```python
from build123d import *

# Parameters (mm, degrees)
SKETCH1_R           = 41.148
BOSS_EXTRUDE1_DEPTH = 38.1
SKETCH2_R           = 3.18135
CUT_EXTRUDE1_DEPTH  = 29.464
CIRPATTERN1_COUNT   = 6
SKETCH3_R           = 44.45
SKETCH3_R_2         = 41.148
BOSS_EXTRUDE2_DEPTH = 57.15
FILLET1_R           = 12.7
CHAMFER1_SIZE       = 1.27
CHAMFER1_SIZE2      = 0.592210726


with BuildPart() as part:
    # Sketch1 → Boss-Extrude1 (new body)
    with BuildSketch(Plane(origin=(0, 0, 0), x_dir=(1, 0, 0), z_dir=(0, 1, 0))):
        Polygon((0, -58.65878735), (50.8, -29.329393675), (50.8, 29.329393675), (0, 58.65878735), (-50.8, 29.329393675), (-50.8, -29.329393675), align=None)
        with Locations(Location((0, 0, 0), (0, 0, 90))):
            Circle(SKETCH1_R, mode=Mode.SUBTRACT)
    extrude(amount=BOSS_EXTRUDE1_DEPTH)

    # Sketch2 → Cut-Extrude1 (cut)
    with BuildSketch(Plane.ZY.offset(50.8)):
        with Locations((0, 19.05)):
            Circle(SKETCH2_R)
    cut_extrude1 = extrude(amount=-CUT_EXTRUDE1_DEPTH, mode=Mode.SUBTRACT)

    # CirPattern1: Cut-Extrude1 ×6 about axis
    cirpattern1_axis = Axis((0, 38.1, 0), (0, 1, 0))
    for i in range(1, CIRPATTERN1_COUNT):
        add(cut_extrude1.rotate(cirpattern1_axis, i * 360 / CIRPATTERN1_COUNT), mode=Mode.SUBTRACT)

    # Sketch3 → Boss-Extrude2 (add)
    with BuildSketch(Plane(origin=(-50.8, 38.1, -29.329393675), x_dir=(1, 0, 0), z_dir=(0, -1, 0))):
        with Locations(Location((50.8, 29.329393675, 0), (0, 0, 270))):
            Circle(SKETCH3_R)
        with Locations(Location((50.8, 29.329393675, 0), (0, 0, 270))):
            Circle(SKETCH3_R_2, mode=Mode.SUBTRACT)
    extrude(amount=-BOSS_EXTRUDE2_DEPTH)

    # Fillet1
    fillet1_edges = [part.edges().sort_by_distance(p)[0] for p in [
        (-50.8, 19.05, 29.329393675),
        (-50.8, 19.05, -29.329393675),
        (0, 19.05, -58.65878735),
        (50.8, 19.05, -29.329393675),
        (50.8, 19.05, 29.329393675),
        (0, 19.05, 58.65878735),
    ]]
    fillet(fillet1_edges, radius=FILLET1_R)

    # Chamfer1
    chamfer1_edges = [part.edges().sort_by_distance(p)[0] for p in [
        (0, 0, 41.148),
        (0, 95.25, 41.148),
    ]]
    chamfer1_side = [part.faces().sort_by_distance(p)[0] for p in [
        (0, 47.625, 41.148),
    ]]
    chamfer(chamfer1_edges, length=CHAMFER1_SIZE, length2=CHAMFER1_SIZE2, reference=chamfer1_side[0])


solid = part.part
```
Part model, mm, in its own coordinate system. Give positions to 0.01 mm unless a question says otherwise; leave off trailing zeros. Order: outer loops, then holes, each group sorted by start corner. A loop starts at its lowest first (then second) coordinate and runs counter-clockwise, first axis right, second up. Notation, with made-up numbers: (82.5, 44.25) - (118.5, 44.25) arc R26 ccw to (118.5, 77.25) - close; hole circle Ø3 at (30, -32). An arc over 180 degrees is marked (long way). Use one line per item in the form item = value.
Item 1: Probe probe 1 along Z at (x, y) = (44.5, 19.05); probe 2 along Y at (x, z) = (48, 0); probe 3 along Z at (x, y) = (-24.5, 86). List the from-to ranges inside material, lowest first. Write a range as from..to.
Solution:
probe_1 = -32.97..-3.18, 3.18..32.97
probe_2 = 0..15.87, 22.23..38.1
probe_3 = -37.09..-33.06, 33.06..37.09
Item 2: Slice it at A-A on y = 10. Give the cut face in (x, z), and give its area (3 significant figures).
Solution:
outline = (-50.8, -22) arc R12.7 ccw to (-44.45, -33) - (-6.35, -54.99) arc R12.7 ccw to (6.35, -54.99) - (44.45, -33) arc R12.7 ccw to (50.8, -22) - (50.8, 22) arc R12.7 ccw to (44.45, 33) - (6.35, 54.99) arc R12.7 ccw to (-6.35, 54.99) - (-44.45, 33) arc R12.7 ccw to (-50.8, 22) - close; hole circle Ø82.3 at (0, 0)
area = 3,570 mm2
Item 3: Two-plate mould, pull along Z, no slides. Class faces 1 (the face through (37.48, 66.27, -23.9)), 2 (the face through (49.05, 19.32, 28.43)), 3 (the face through (25.67, 23.02, -43.84)), 4 (the face through (-40.798, 46.976, 5.357)): released by +Z, released by -Z, zero draft, split by the parting line, or undercut.
Solution:
face_1 = split by the parting line
face_2 = released by +Z
face_3 = released by -Z
face_4 = undercut
Item 4: Pin check, flat tips, straight feed: pin 1 Ø6 at (y, z) = (75, 20.5) entering from +X; pin 2 Ø12 at (x, z) = (19, -34.5) entering from +Y; pin 3 Ø4 at (y, z) = (47.5, 15.5) entering from -X; pin 4 Ø6 at (y, z) = (80.5, -8) entering from -X. Stop position of each tip, or through.
Solution:
pin_1 = 40.86
pin_2 = 95.25
pin_3 = -42.35
pin_4 = -44.17
Item 5: Slice it at D-D on y = 20.5. Count the separate pieces of the cut face and the enclosed holes in it, and give its area (3 significant figures).
Solution:
separate_pieces = 6
enclosed_holes = 0
area = 3,240 mm2
Item 6: Slice it at B-B on x = 0. Give the cut face in (y, z), and give its area (3 significant figures).
Solution:
outline = (0, -56.69) - (38.1, -56.69) - (38.1, -44.45) - (95.25, -44.45) - (95.25, -41.74) - (93.98, -41.15) - (1.27, -41.15) - (0, -41.74) - close; (0, 41.74) - (1.27, 41.15) - (93.98, 41.15) - (95.25, 41.74) - (95.25, 44.45) - (38.1, 44.45) - (38.1, 56.69) - (0, 56.69) - close
area = 1,560 mm2
Item 7: Slice it at C-C on y = 54. Give the cut face in (x, z), and give its area (3 significant figures).
Solution:
outline = circle Ø88.9 at (0, 0); hole circle Ø82.3 at (0, 0)
area = 888 mm2
